Geometry check sheet. Reference: drawing and pictorial views, mm from the part's lowest x, y, z. Coordinates: 2 decimals unless noted, no trailing zeros. Loops run counter-clockwise (first coordinate to the right, second up) from the corner with the lowest first, then second, coordinate; pieces in that order, holes last. Notation, with made-up numbers: (39, 31) -> (91, 31) arc R10 ccw to (91, 39) -> close; hole circle Ø9 at (77, 89.5). An arc over 180 degrees is marked (long way). Answer as a JSON object with one key per item and string values. Group by question number.
Q1. Cross-section at C-C on z = 13. Record the boundary of the cut face in (x, y) (1 decimal).
Q2. Cross-section at A-A on x = 32.5. Record the boundary of the cut face in (y, z).
Q3. Scan lines: L1, parallel to Z at x = 34, y = 1.75; L2, parallel to Z at x = 35.5, y = 1.5 (1 decimal); L3, parallel to X at y = 0.85, z = 30.5 (1 decimal). Record each from-to range of solid material in increasing order.
Q4. Gauge pin test, flat end, axial feed: pin 1 Ø0.6 at (y, z) = (1, 25) entering from +X. Record the tip position at first contact, or that the pin passes through.
Q5. Cross-section at D-D on x = 12. Record the boundary of the cut face in (y, z).
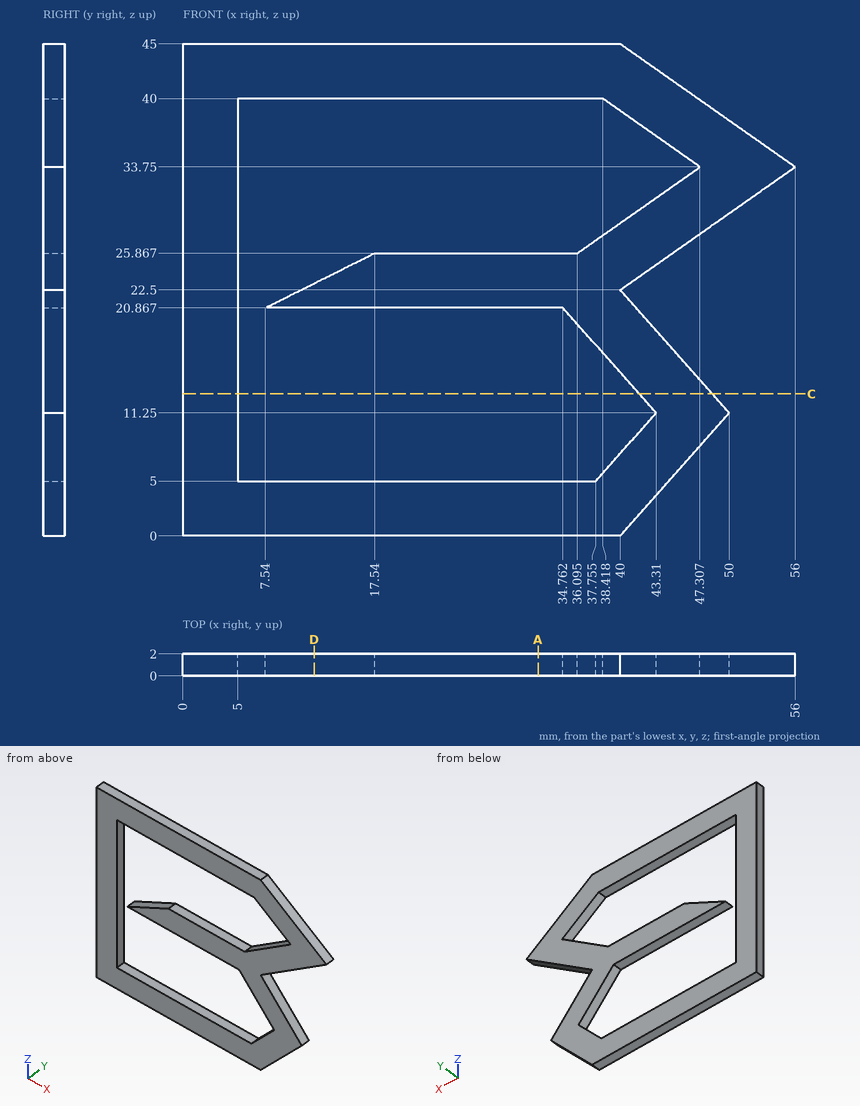
Computed values:
{
 "1": {"outline": "(0, 0) -> (5, 0) -> (5, 2) -> (0, 2) -> close; (41.8, 0) -> (48.4, 0) -> (48.4, 2) -> (41.8, 2) -> close"},
 "2": {"outline": "(0, 0) -> (2, 0) -> (2, 5) -> (0, 5) -> close; (0, 20.87) -> (2, 20.87) -> (2, 25.87) -> (0, 25.87) -> close; (0, 40) -> (2, 40) -> (2, 45) -> (0, 45) -> close"},
 "3": {"L1": "z = 0 to 5, 20.87 to 25.87, 40 to 45", "L2": "z = 0 to 5, 20 to 25.9, 40 to 45", "L3": "x = 0 to 5, 42.7 to 51.4"},
 "4": {"pin 1": "stops at x = 43.98"},
 "5": {"outline": "(0, 0) -> (2, 0) -> (2, 5) -> (0, 5) -> close; (0, 20.87) -> (2, 20.87) -> (2, 23.1) -> (0, 23.1) -> close; (0, 40) -> (2, 40) -> (2, 45) -> (0, 45) -> close"}
}
